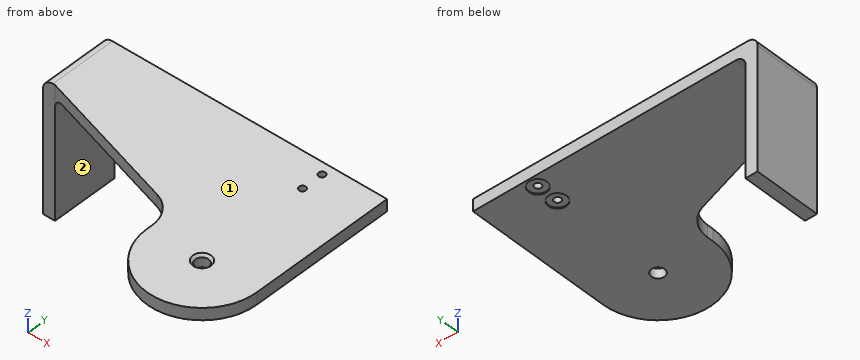
from build123d import *

# Parameters (mm, degrees)
ESTRUSIONE_ESTRUSIONE1_DEPTH                 = 6
SCHIZZO3_W                                   = 136.2
SCHIZZO3_H                                   = 72.5
ESTRUSIONE_ESTRUSIONE2_DEPTH                 = 6
TAGLIO_ESTRUSIONE1_DEPTH                     = 131.797324132
RACCORDO5_R                                  = 15
ESTRUSIONE_ESTRUSIONE5_DEPTH                 = 6
ESTRUSIONE_ESTRUSIONE5_DEPTH_BACK            = 60
SCHIZZO9_W                                   = 6
SCHIZZO9_H                                   = 33.15279029
RACCORDO6_R                                  = 5
RACCORDO7_R                                  = 5
FORO_FILETTATO_G1_16_1_D                     = 6.6
FORO_FILETTATO_G1_16_1_CSINK_D               = 9.05
FORO_FILETTATO_G1_16_1_CSINK_ANGLE           = 90
FORO_LAMATO_PER_BULLONE_M3_A_TESTA_E_2_COUNT = 2
FORO_LAMATO_PER_BULLONE_M3_A_TESTA_E_2_PITCH = 10.95


with BuildPart() as part:
    # Schizzo2 → Estrusione-Estrusione1 (new body)
    with BuildSketch(Plane.XY):
        with BuildLine():
            Line((-27.5, 0), (-27.5, 45))
            ThreePointArc((-27.5, 45), (0, 72.5), (27.5, 45))
            Line((27.5, 45), (27.5, 0))
            ThreePointArc((27.5, 0), (0, -27.5), (-27.5, 0))
        make_face()
    extrude(amount=ESTRUSIONE_ESTRUSIONE1_DEPTH)

    # Schizzo3 → Estrusione-Estrusione2 (add)
    with BuildSketch(Plane.XY):
        with Locations((-40.6, 36.25)):
            Rectangle(SCHIZZO3_W, SCHIZZO3_H)
    extrude(amount=ESTRUSIONE_ESTRUSIONE2_DEPTH)

    # Schizzo4 → Taglio-Estrusione1 (cut, through all)
    with BuildSketch(Plane.XY.offset(6)):
        Polygon((-27.5, 0), (-108.7, 0), (-108.7, 39.34720971), (-27.5, 14.142426235), align=None)
    extrude(amount=-TAGLIO_ESTRUSIONE1_DEPTH, mode=Mode.SUBTRACT)

    # Raccordo5
    raccordo5_edges = [part.edges().sort_by_distance(p)[0] for p in [
        (-27.5, 14.142426235, 3),
    ]]
    fillet(raccordo5_edges, radius=RACCORDO5_R)

    # Schizzo9 → Estrusione-Estrusione5 (add, two sides: drawn at the far end of the back side and taken through both)
    with BuildSketch(Plane.XY.offset(-ESTRUSIONE_ESTRUSIONE5_DEPTH_BACK)):
        with Locations((-111.7, 55.923604855)):
            Rectangle(SCHIZZO9_W, SCHIZZO9_H)
    extrude(amount=ESTRUSIONE_ESTRUSIONE5_DEPTH + ESTRUSIONE_ESTRUSIONE5_DEPTH_BACK)

    # Raccordo6
    raccordo6_edges = [part.edges().sort_by_distance(p)[0] for p in [
        (-108.7, 55.923604855, 0),
    ]]
    fillet(raccordo6_edges, radius=RACCORDO6_R)

    # Raccordo7
    raccordo7_edges = [part.edges().sort_by_distance(p)[0] for p in [
        (-114.7, 55.923604855, 6),
    ]]
    fillet(raccordo7_edges, radius=RACCORDO7_R)

    # Foro filettato G1/16-1 (through all)
    with Locations(Plane.XY.offset(6)):
        with Locations((0, 0)):
            CounterSinkHole(FORO_FILETTATO_G1_16_1_D / 2, FORO_FILETTATO_G1_16_1_CSINK_D / 2, counter_sink_angle=FORO_FILETTATO_G1_16_1_CSINK_ANGLE)

    # Schizzo20 → Foro lamato per Bullone M3 a testa esagonale-3 (revolve, cut)
    with BuildSketch(Plane(origin=(0, 67, 0), x_dir=(0, 1, 0), z_dir=(1, 0, 0))):
        Polygon((0, 0), (0, 6), (1.7, 6), (1.7, 0.5), (4.5, 0.5), (4.5, 0.025), (4.525, 0), align=None)
    foro_lamato_per_bullone_m3_a_testa_esago = revolve(axis=Axis((0, 67, -6.35), (0, 0, 1)), mode=Mode.SUBTRACT)

    # Foro lamato per Bullone M3 a testa e 2: Foro lamato per Bullone M3 a testa esagonale-3 ×2
    with Locations(*[(0, -i * FORO_LAMATO_PER_BULLONE_M3_A_TESTA_E_2_PITCH, 0) for i in range(1, FORO_LAMATO_PER_BULLONE_M3_A_TESTA_E_2_COUNT)]):
        add(foro_lamato_per_bullone_m3_a_testa_esago, mode=Mode.SUBTRACT)


solid = part.part
CAD build for the part. Positions are in the model's coordinates, mm. Face numbers are marked on the shaded views. A direction names the side the tool comes from. Give positions to 0.01 mm unless a question says otherwise; leave off trailing zeros. Loops run counter-clockwise (first coordinate to the right, second up) from the corner with the lowest first, then second, coordinate; pieces in that order, holes last. Notation, with made-up numbers: M 13,38.5 L 36,38.5 A17 ccw 36,68.5 Z; hole C 30.25,84 d3. An arc over 180 degrees is marked long. One line per question, with ' | ' between items. Start each with the question number.
1. Saw through at B-B on y = 56.05. Give the cut face in (x, z) (3 decimals).
2. Saw through at D-D on x = -66. Give the cut face in (y, z).
3. Saw through at A-A on x = 0. State how many separate pieces and enclosed holes the cut face has, plus the area to 3 significant figures.
4. Saw through at C-C on z = -14.5. Give the cut face in (x, y).
5. 3-axis set-ups, long thin cutter, end or side, ignore diameter. For the marked faces 1 and 2: which of +Z, -Z, +X, -X, +Y, -Y reach the whole face in a straight line?
6. Probe L1, parallel to Y at x = 0, z = 2; L2, parallel to Y at x = 0, z = 0.4; L3, parallel to Z at x = -26.5, y = 21. List the from-to ranges inside material, lowest first. Write a range as from..to.
7. Flat gauge pins, fed straight in: pin 1 (10.5 mm diameter, centred on x = 0, y = 56.05, fed in from +Z); pin 2 (2 mm diameter, centred on x = 0, y = 67, fed in from -Z); pin 3 (6.5 mm diameter, centred on x = -112, z = -38.5, fed in from -Y); pin 4 (8.5 mm diameter, centred on x = 0, y = 0, fed in from -Z). Where does each tip first touch, or does it go through?
Result sheet:
1) outline: M -114.7,-60 L -108.7,-60 L -108.7,-5 A5 cw -103.7,0 L -4.525,0 L -4.5,0.025 L -4.5,0.5 L -1.7,0.5 L -1.7,6 L -109.7,6 A5 ccw -114.7,1 Z; M 1.7,0.5 L 4.5,0.5 L 4.5,0.025 L 4.525,0 L 27.5,0 L 27.5,6 L 1.7,6 Z
2) outline: M 26.09,0 L 72.5,0 L 72.5,6 L 26.09,6 Z
3) separate pieces: 4 | enclosed holes: 0 | area: 512 mm^2
4) outline: M -114.7,39.35 L -108.7,39.35 L -108.7,72.5 L -114.7,72.5 Z
5) face 1: +Z, +X, -X, +Y, -Y | face 2: -Z, +X, +Y, -Y
6) L1: y = -27.5..-3.3, 3.3..54.35, 57.75..65.3, 68.7..72.5 | L2: y = -27.5..-3.3, 3.3..51.55, 60.55..62.5, 71.5..72.5 | L3: z = 0..6
7) pin 1: stops at z = 6 | pin 2: passes through | pin 3: stops at y = 39.35 | pin 4: stops at z = 0
